Check sheet for the modelled part. Datum: model origin and axes. Units: mm. A direction names the side the tool comes from. Coordinates: 2 decimals unless noted, no trailing zeros. Write each loop counter-clockwise with the first axis right and the second up, starting at its lowest first coordinate (ties: lowest second). Pieces come first, ordered by that corner, then holes. Notation, with made-up numbers: (75, -29) - (100, -29) arc R18 ccw to (100, -11) - close; hole circle Ø6 at (41.5, 76.25). An arc over 180 degrees is marked (long way). Write each question's results on one line, items separated by ' | '.
Autodesk Inventor part; units mm, degrees
ref_plane "YZ Plane" through (0, 0, 0) normal (1, 0, 0) x (0, 1, 0)
ref_plane "XZ Plane" through (0, 0, 0) normal (0, 1, 0) x (-1, 0, 0)
ref_plane "XY Plane" through (0, 0, 0) normal (0, 0, 1) x (1, 0, 0)
sketch "Sketch1" plane through (0, 0, 0) normal (0, 1, 0) x (-1, 0, 0)
  line L0 (85, 49) -> (-85, 49)
  line L1 (-85, 49) -> (-85, -49)
  line L2 (-85, -49) -> (85, -49)
  line L3 (85, -49) -> (85, 49)
  line L4 (85, 49) -> (-85, -49) construction
  line L5 (-85, 49) -> (85, -49) construction
  circle A0 centre (80, -44) radius 1.7
  circle A1 centre (80, 44) radius 1.7
  circle A2 centre (-80, -44) radius 1.7
  circle A3 centre (-80, 44) radius 1.7
  circle A4 centre (50, -44) radius 1.7
  circle A5 centre (50, 44) radius 1.7
  point P0 (0, 0)
  dimension "d0" = 170
  dimension "d1" = 98
  dimension "d2" = 5
  dimension "d3" = 5
  dimension "d4" = 3.4
  dimension "d7" = 88
  dimension "d10" = 160
  dimension "d25" = 30
extrude "Extrusion1" add sketch "Sketch1" along normal blind 4
fillet "Fillet1" radius 5 4 edges at (85, 2, 49) (85, 2, -49) (-85, 2, 49) (-85, 2, -49)
sketch "Sketch2" plane through (0, 4, 0) normal (0, 1, 0) x (1, 0, 0)
  line L0 (-85, 44) -> (-85, -44)
  line L1 (-72, -33.5) -> (-62, -33.5)
  line L2 (-72, -37.5) -> (-72, -33.5)
  line L3 (-72, -23.5) -> (-72, -37.5)
  line L4 (18, 33.5) -> (10, 33.5)
  line L5 (10, 33.5) -> (10, 25.5)
  line L6 (10, 25.5) -> (18, 25.5)
  line L7 (18, 25.5) -> (18, 33.5)
  line L8 (10, 25.5) -> (22, 25.5)
  line L9 (22, 25.5) -> (22, 37.5)
  line L10 (22, 37.5) -> (10, 37.5)
  line L11 (10, 37.5) -> (10, 25.5)
  line L12 (-72, -33.5) -> (-64, -33.5)
  line L13 (-64, -33.5) -> (-64, -25.5)
  line L14 (-64, -25.5) -> (-72, -25.5)
  line L15 (-72, -25.5) -> (-72, -33.5)
  line L16 (-64, -25.5) -> (-76, -25.5)
  line L17 (-76, -25.5) -> (-76, -37.5)
  line L18 (-76, -37.5) -> (-64, -37.5)
  line L19 (-64, -37.5) -> (-64, -25.5)
  line L20 (-25.0039, 0) -> (-47.7766, 0)
  line L21 (-72, 33.5) -> (-62, 33.5)
  line L22 (-72, 37.5) -> (-72, 33.5)
  line L23 (-72, 23.5) -> (-72, 37.5)
  line L24 (18, -33.5) -> (10, -33.5)
  line L25 (10, -33.5) -> (10, -25.5)
  line L26 (10, -25.5) -> (18, -25.5)
  line L27 (18, -25.5) -> (18, -33.5)
  line L28 (10, -25.5) -> (22, -25.5)
  line L29 (22, -25.5) -> (22, -37.5)
  line L30 (22, -37.5) -> (10, -37.5)
  line L31 (10, -37.5) -> (10, -25.5)
  line L32 (-72, 33.5) -> (-64, 33.5)
  line L33 (-64, 33.5) -> (-64, 25.5)
  line L34 (-64, 25.5) -> (-72, 25.5)
  line L35 (-72, 25.5) -> (-72, 33.5)
  line L36 (-64, 25.5) -> (-76, 25.5)
  line L37 (-76, 25.5) -> (-76, 37.5)
  line L38 (-76, 37.5) -> (-64, 37.5)
  line L39 (-64, 37.5) -> (-64, 25.5)
  point P0 (0, 0)
  point P1 (10, 33.5)
  point P2 (18, 25.5)
  dimension "d30" = 13
  dimension "d31" = 33.5
  dimension "d36" = 67
  dimension "d37" = 90
  dimension "d38" = 8
  dimension "d39" = 8
  dimension "d40" = 12
  dimension "d41" = 12
  dimension "d44" = 8
  dimension "d45" = 8
  dimension "d46" = 12
  dimension "d47" = 12
extrude "Extrusion2" cut sketch "Sketch2" against normal through all contours L1 L19 L18 L2 | L2 L18 L17 L16 L3 | L4 L11 L10 L9 L8 L7 | L22 L38 L39 L21 | L23 L36 L37 L38 L22 | L27 L28 L29 L30 L31 L24
sketch "Sketch3" plane through (0, 4, 0) normal (0, 1, 0) x (1, 0, 0)
  line L0 (-64, -33.5) -> (-64, -37.5)
  line L1 (-64, -37.5) -> (-76, -37.5)
  line L2 (-76, -37.5) -> (-76, -25.5)
  line L3 (-76, -25.5) -> (-72, -25.5)
  line L4 (-72, -25.5) -> (-72, -33.5)
  line L5 (-72, -33.5) -> (-64, -33.5)
  line L6 (18, -25.5) -> (22, -25.5)
  line L7 (22, -25.5) -> (22, -37.5)
  line L8 (22, -37.5) -> (10, -37.5)
  line L9 (10, -37.5) -> (10, -33.5)
  line L10 (10, -33.5) -> (18, -33.5)
  line L11 (18, -33.5) -> (18, -25.5)
  line L12 (18, 33.5) -> (10, 33.5)
  line L13 (10, 33.5) -> (10, 37.5)
  line L14 (10, 37.5) -> (22, 37.5)
  line L15 (22, 37.5) -> (22, 25.5)
  line L16 (22, 25.5) -> (18, 25.5)
  line L17 (18, 25.5) -> (18, 33.5)
  line L18 (-76, 25.5) -> (-76, 37.5)
  line L19 (-76, 37.5) -> (-64, 37.5)
  line L20 (-64, 37.5) -> (-64, 33.5)
  line L21 (-64, 33.5) -> (-72, 33.5)
  line L22 (-72, 33.5) -> (-72, 25.5)
  line L23 (-72, 25.5) -> (-76, 25.5)
  arc A0 (-80, 49) -> (-85, 44) centre (-80, 44) ccw
  line L24 (-85, 44) -> (-85, -44)
  arc A1 (-85, -44) -> (-80, -49) centre (-80, -44) ccw
  line L25 (-80, -49) -> (80, -49)
  arc A2 (80, -49) -> (85, -44) centre (80, -44) ccw
  line L26 (85, -44) -> (85, 44)
  arc A3 (85, 44) -> (80, 49) centre (80, 44) ccw
  line L27 (80, 49) -> (-80, 49)
  circle A4 centre (-80, 44) radius 1.7
  circle A5 centre (-80, -44) radius 1.7
  circle A6 centre (80, 44) radius 1.7
  circle A7 centre (80, -44) radius 1.7
  circle A8 centre (-50, 44) radius 1.7
  circle A9 centre (-50, -44) radius 1.7
  point P0 (0, 0)
equation "\"d39\" = d38"
equation "\"d41\" = d40"
equation "\"d44\" = d39"
equation "\"d45\" = d44"
equation "\"d46\" = d41"
equation "\"d47\" = d41"
properties part number "upper_plate" material "MDF Medium Density Fiberboard"
1. Material ranges on L1, parallel to X at y = 0.75, z = 31; L2, parallel to Z at x = -50, y = 2.75; L3, parallel to X at y = 2.8, z = 35, recorded low to high. Write a range as [from, to].
Values follow:
L1: x = [-85, -76], [-72, 18], [22, 85] | L2: z = [-49, -45.7], [-42.3, 42.3], [45.7, 49] | L3: x = [-85, -76], [-64, 10], [22, 85]
2. Sectioned sample at C-C (y = 2.8). Give the number of separate pieces and of enclosed holes in the cut face, then the cut area to 3 significant figures.
Values follow:
separate pieces: 1 | enclosed holes: 10 | area: 16,300 mm^2
3. Draft check along Z on faces 1 (the flat face through (1, 2, -49)), 2 (the cylindrical face through (81.7, 1.97, -44.07)), 3 (the flat face through (16, 2, -37.5)), 4 (the flat face through (-1, 2, 49)). Enter one of: pulls with the +Z half, pulls with the -Z half, needs draft (parallel to the pull), parting line crosses it, or undercut.
Values follow:
face 1: pulls with the -Z half | face 2: undercut | face 3: undercut | face 4: pulls with the +Z half
4. Access from +Z, -Z, +X, -X, +Y, -Y to the whole of each face (thin tool, end or side, straight path). Record for faces 5 (the cylindrical face through (84, 2, -47)), 6 (the flat face through (20, 2, -25.5)).
Values follow:
face 5: -Z, +X, +Y, -Y | face 6: +Y, -Y
5. Go/stop test with a flat-tipped pin: pin 1 (3 mm diameter, centred on x = -50, z = -44, fed in from -Y). Record where the tip stops, or that it passes through.
Values follow:
pin 1: passes through
6. Sectioned sample at B-B (z = 28.5). Record the cut outline in (x, y), then the cut area to 3 significant figures.
Values follow:
outline: (-85, 0) - (-76, 0) - (-76, 4) - (-85, 4) - close; (-72, 0) - (18, 0) - (18, 4) - (-72, 4) - close; (22, 0) - (85, 0) - (85, 4) - (22, 4) - close | area: 648 mm^2
7. Sectioned sample at A-A (x = -50). Record the cut outline in (y, z), then the cut area to 3 significant figures.
Values follow:
outline: (0, -49) - (4, -49) - (4, -45.7) - (0, -45.7) - close; (0, -42.3) - (4, -42.3) - (4, 42.3) - (0, 42.3) - close; (0, 45.7) - (4, 45.7) - (4, 49) - (0, 49) - close | area: 365 mm^2
